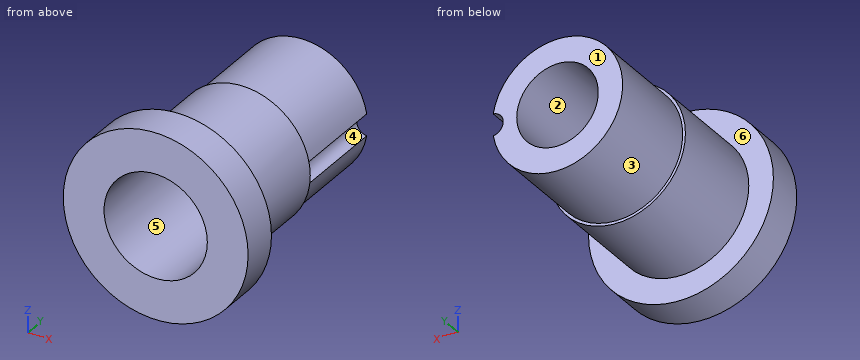
from build123d import *

# Parameters (mm, degrees)
SKETCH2_R          = 3.175
CUT_EXTRUDE1_DEPTH = 28.575


with BuildPart() as part:
    # Sketch1 → Revolve1 (revolve)
    with BuildSketch(Plane.XY):
        with BuildLine():
            Line((15.08125, -34.925), (26.9875, -34.925))
            Line((26.9875, -34.925), (26.9875, -23.8125))
            Line((26.9875, -23.8125), (19.812, -23.8125))
            Line((19.812, -23.8125), (19.812, 6.35))
            Line((19.812, 6.35), (19.0246, 6.35))
            Line((19.0246, 6.35), (19.0246, 34.925))
            Line((19.0246, 34.925), (11.90625, 34.925))
            Line((11.90625, 34.925), (11.90625, 3.175))
            ThreePointArc((11.90625, 3.175), (14.15131403, 2.24506403), (15.08125, 0))
            Line((15.08125, 0), (15.08125, -34.925))
        make_face()
    revolve(axis=Axis((0, -34.925, 0), (0, 1, 0)))

    # Sketch2 → Cut-Extrude1 (cut)
    with BuildSketch(Plane(origin=(0, 34.925, 0), x_dir=(1, 0, 0), z_dir=(0, 1, 0))):
        with Locations((19.0246, 0)):
            Circle(SKETCH2_R)
    extrude(amount=-CUT_EXTRUDE1_DEPTH, mode=Mode.SUBTRACT)


solid = part.part
Build history of the part. All positions in model axes, mm. Face numbers are marked on the shaded views. A direction names the side the tool comes from. Coordinates: 2 decimals unless noted, no trailing zeros. Order: outer loops, then holes, each group sorted by start corner. A loop starts at its lowest first (then second) coordinate and runs counter-clockwise, first axis right, second up. Notation, with made-up numbers: (53.25, 47.5) - (79.25, 47.5) arc R19 ccw to (79.25, 60.5) - close; hole circle Ø2 at (84, 32). An arc over 180 degrees is marked (long way). Write each question's results on one line, items separated by ' | '. Start each with the question number.
Item 1: Wall check: probe 1 along Z at (x, y) = (0, 11); probe 2 along X at (y, z) = (-26, 0); probe 3 along Z at (x, y) = (0, -23.5). Give the ranges that are in metal, low to high. Write a range as [from, to].
Item 2: Band-saw the part on D-D on y = -5. Write the cut outline in (x, z), and give its area (3 significant figures).
Item 3: Tool access for the marked faces 4, 5 and 6: list every direction of +Z, -Z, +X, -X, +Y, -Y with a clear straight run to the whole face (end or side of a thin tool).
Item 4: Mould opens along Z. For the marked faces 1, 2 and 3 say: released by +Z, released by -Z, zero draft, split by the parting line, or undercut.
Item 5: Flat gauge pins, fed straight in: pin 1 (5 mm diameter, centred on x = 8, y = -16.5, fed in from +Z); pin 2 (5 mm diameter, centred on x = 20.5, z = 12, fed in from +Y); pin 3 (3 mm diameter, centred on y = 17, z = -1, fed in from +X). Where does each tip first touch, or does it go through?
Numbers:
1) probe 1: [-19.02, -11.91], [11.91, 19.02] | probe 2: [-26.99, -15.08], [15.08, 26.99] | probe 3: [-19.81, -15.08], [15.08, 19.81]
2) outline: circle Ø39.62 at (0, 0); hole circle Ø30.16 at (0, 0) | area: 519 mm^2
3) face 4: +X, +Y | face 5: -Y | face 6: +Y
4) face 1: zero draft | face 2: undercut | face 3: split by the parting line
5) pin 1: z = 19.03 | pin 2: y = -23.81 | pin 3: x = 17.07
